Check sheet for the drawn part. Datum: minimum x, y, z corner. Units: mm. A direction names the side the tool comes from. Round coordinates to 2 decimals unless told otherwise and drop trailing zeros. Loops run counter-clockwise (first coordinate to the right, second up) from the corner with the lowest first, then second, coordinate; pieces in that order, holes last.
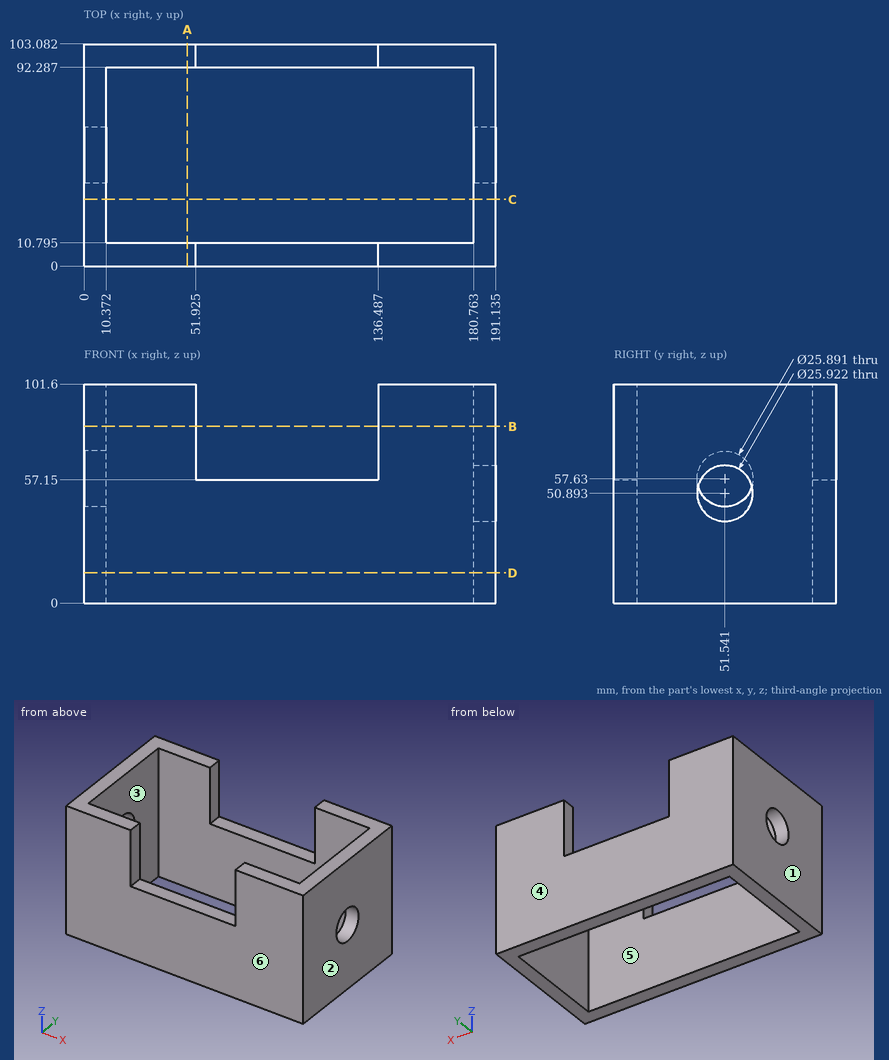
1) Gauge pin test, flat ends, axial feed: pin 1 (20.5 mm diameter, centred on y = 51.54, z = 57.63, fed in from -X); pin 2 (8 mm diameter, centred on y = 21, z = 48, fed in from -X); pin 3 (3 mm diameter, centred on x = 119.5, y = 13, fed in from -Z); pin 4 (8.5 mm diameter, centred on x = 111, y = 4, fed in from +Z). Record the tip position at first contact, or that the pin passes through.
Report:
pin 1: stops at x = 180.76
pin 2: stops at x = 0
pin 3: passes through
pin 4: stops at z = 57.15
2) Access from +Z, -Z, +X, -X, +Y, -Y to the whole of each face (thin tool, end or side, straight path). Record for the marked faces 5 and 6.
Report:
face 5: +Z, -Z
face 6: +Z, -Z, +X, -X, -Y
3) Sectioned sample at C-C, the plane y = 31. Record the cut outline in (x, z) (1 decimal), then the cut area to 3 significant figures.
Report:
outline: (0, 0) - (10.4, 0) - (10.4, 101.6) - (0, 101.6) - close; (180.8, 0) - (191.1, 0) - (191.1, 101.6) - (180.8, 101.6) - close
area: 2,110 mm2
4) Sectioned sample at D-D, the plane z = 14. Record the cut outline in (x, y) (1 decimal), then the cut area to 3 significant figures.
Report:
outline: (0, 0) - (191.1, 0) - (191.1, 103.1) - (0, 103.1) - close; hole (10.4, 10.8) - (180.8, 10.8) - (180.8, 92.3) - (10.4, 92.3) - close
area: 5,820 mm2
5) Mould release check, pull along X, two halves, no side actions. Record for the marked faces 1, 2, 3 and 4: +X half, -X half, draft (parallel to the pull), parting line (faces both ways), or undercut.
Report:
face 1: -X half
face 2: +X half
face 3: undercut
face 4: draft
6) Sectioned sample at A-A, the plane x = 48. Record the cut outline in (y, z) (1 decimal).
Report:
outline: (0, 0) - (10.8, 0) - (10.8, 101.6) - (0, 101.6) - close; (92.3, 0) - (103.1, 0) - (103.1, 101.6) - (92.3, 101.6) - close
7) Scan lines: line 1 along X through (y, z) = (35.5, 24) (1 decimal); line 2 along Y through (x, z) = (35, 13) (1 decimal); line 3 along X through (y, z) = (8, 63.5) (1 decimal). Record each from-to range of solid material in increasing order.
Report:
line 1: x = 0 to 10.4, 180.8 to 191.1
line 2: y = 0 to 10.8, 92.3 to 103.1
line 3: x = 0 to 51.9, 136.5 to 191.1
8) Sectioned sample at B-B, the plane z = 82. Record the cut outline in (x, y) (1 decimal).
Report:
outline: (0, 0) - (51.9, 0) - (51.9, 10.8) - (10.4, 10.8) - (10.4, 92.3) - (51.9, 92.3) - (51.9, 103.1) - (0, 103.1) - close; (136.5, 0) - (191.1, 0) - (191.1, 103.1) - (136.5, 103.1) - (136.5, 92.3) - (180.8, 92.3) - (180.8, 10.8) - (136.5, 10.8) - close
